Source: CAD feature listing. Evaluate the final solid. Frame: model axes, mm. A direction names the side the tool comes from. Give positions to 0.01 mm unless a question says otherwise; leave off trailing zeros. Order: outer loops, then holes, each group sorted by start corner. A loop starts at its lowest first (then second) coordinate and runs counter-clockwise, first axis right, second up.
from build123d import *

# Parameters (mm, degrees)
PAD_DEPTH       = 20
SKETCH004_R     = 2
POCKET002_DEPTH = 157.001
SKETCH005_R     = 2
POCKET003_DEPTH = 85.001


with BuildPart() as part:
    # Sketch → Pad (new body)
    with BuildSketch(Plane.XY):
        Polygon((-10, -42.5), (147, -42.5), (147, -30.5), (0, -30.5), (0, 30.5), (147, 30.5), (147, 42.5), (-10, 42.5), (-10, 38.5), (-17, 38.5), (-17, 33.5), (-10, 33.5), (-10, -33.5), (-17, -33.5), (-17, -38.5), (-10, -38.5), align=None)
    extrude(amount=PAD_DEPTH)

    # Sketch004 → Pocket002 (cut, through all)
    with BuildSketch(Plane(origin=(-10, 0, 0), x_dir=(0, -1, 0), z_dir=(-1, 0, 0))):
        with Locations((0, 10)):
            Circle(SKETCH004_R)
    extrude(amount=-POCKET002_DEPTH, mode=Mode.SUBTRACT)

    # Sketch005 → Pocket003 (cut, through all)
    with BuildSketch(Plane.XZ.offset(42.5)):
        with Locations((-5, 10)):
            Circle(SKETCH005_R)
        with Locations((137, 10)):
            Circle(SKETCH005_R)
    extrude(amount=-POCKET003_DEPTH, mode=Mode.SUBTRACT)


solid = part.part
1) Section query D-D on z = 2.75. Output: boundary loops of the cut face in (x, y).
Checks:
outline: (-17, -38.5) - (-10, -38.5) - (-10, -42.5) - (147, -42.5) - (147, -30.5) - (0, -30.5) - (0, 30.5) - (147, 30.5) - (147, 42.5) - (-10, 42.5) - (-10, 38.5) - (-17, 38.5) - (-17, 33.5) - (-10, 33.5) - (-10, -33.5) - (-17, -33.5) - close
2) Pull-direction query (Z, two-part tool) for faces 4 (the face through (59, 32, 20)), 5 (the face through (135, 36, 10)), 6 (the face through (70, 42.5, 10)), 7 (the face through (59, 32, 0)); classes: +Z half, -Z half, draft (parallel to the pull), parting line (faces both ways), or undercut.
Checks:
face 4: +Z half
face 5: undercut
face 6: draft
face 7: -Z half
3) First-contact query: pin 1 Ø10 at (x, y) = (70, 21) entering from -Z; pin 2 Ø5 at (y, z) = (0, 10) entering from +X; pin 3 Ø5.5 at (x, z) = (-14.5, 8) entering from +Y; pin 4 Ø1.2 at (y, z) = (-39.5, 5) entering from -X. Flat tips, straight axial feed; report the tip coordinate or a pass-through.
Checks:
pin 1: passes through
pin 2: stops at x = 0
pin 3: stops at y = 38.5
pin 4: stops at x = -10
4) Reachability of faces 1 (the face through (-13, 38.5, 10)), 2 (the face through (-14, 33.5, 10)), 3 (the face through (0, -0.4, 7.6)) from +Z, -Z, +X, -X, +Y, -Y: full face, straight path, thin tool, end or side. Return the list, or none.
Checks:
face 1: +Z, -Z, -X, +Y
face 2: +Z, -Z, -X
face 3: +Z, -Z, +X
5) Section query A-A on x = 90. Output: boundary loops of the cut face in (y, z).
Checks:
outline: (-42.5, 0) - (-30.5, 0) - (-30.5, 20) - (-42.5, 20) - close; (30.5, 0) - (42.5, 0) - (42.5, 20) - (30.5, 20) - close
6) Section query B-B on x = 137. Output: boundary loops of the cut face in (y, z), and give its area (3 significant figures).
Checks:
outline: (-42.5, 0) - (-30.5, 0) - (-30.5, 8) - (-42.5, 8) - close; (-42.5, 12) - (-30.5, 12) - (-30.5, 20) - (-42.5, 20) - close; (30.5, 0) - (42.5, 0) - (42.5, 8) - (30.5, 8) - close; (30.5, 12) - (42.5, 12) - (42.5, 20) - (30.5, 20) - close
area: 384 mm2
7) Section query C-C on y = -23. Output: boundary loops of the cut face in (x, z).
Checks:
outline: (-10, 0) - (0, 0) - (0, 20) - (-10, 20) - close; hole circle Ø4 at (-5, 10)
8) Ray query, L1, parallel to X at y = -11, z = 10; L2, parallel to Z at x = -5, y = 16.5; L3, parallel to Y at x = 42.5, z = 2. Return the intervals inside material, ascending.
Checks:
L1: x = -10 to -7, -3 to 0
L2: z = 0 to 8, 12 to 20
L3: y = -42.5 to -30.5, 30.5 to 42.5
